The figure shows three views and two pictorial views of one solid part (mm, origin at its lowest corner). Answer the questions. A direction names the side the tool comes from. Round coordinates to 2 decimals unless told otherwise and drop trailing zeros. Order: outer loops, then holes, each group sorted by start corner. A loop starts at its lowest first (then second) coordinate and runs counter-clockwise, first axis right, second up. Notation, with made-up numbers: M 29,3.5 L 78,3.5 A13 ccw 78,17.5 Z; hole C 19.25,-32 d4. An arc over 180 degrees is marked long. Answer as CSV lines item,"result".
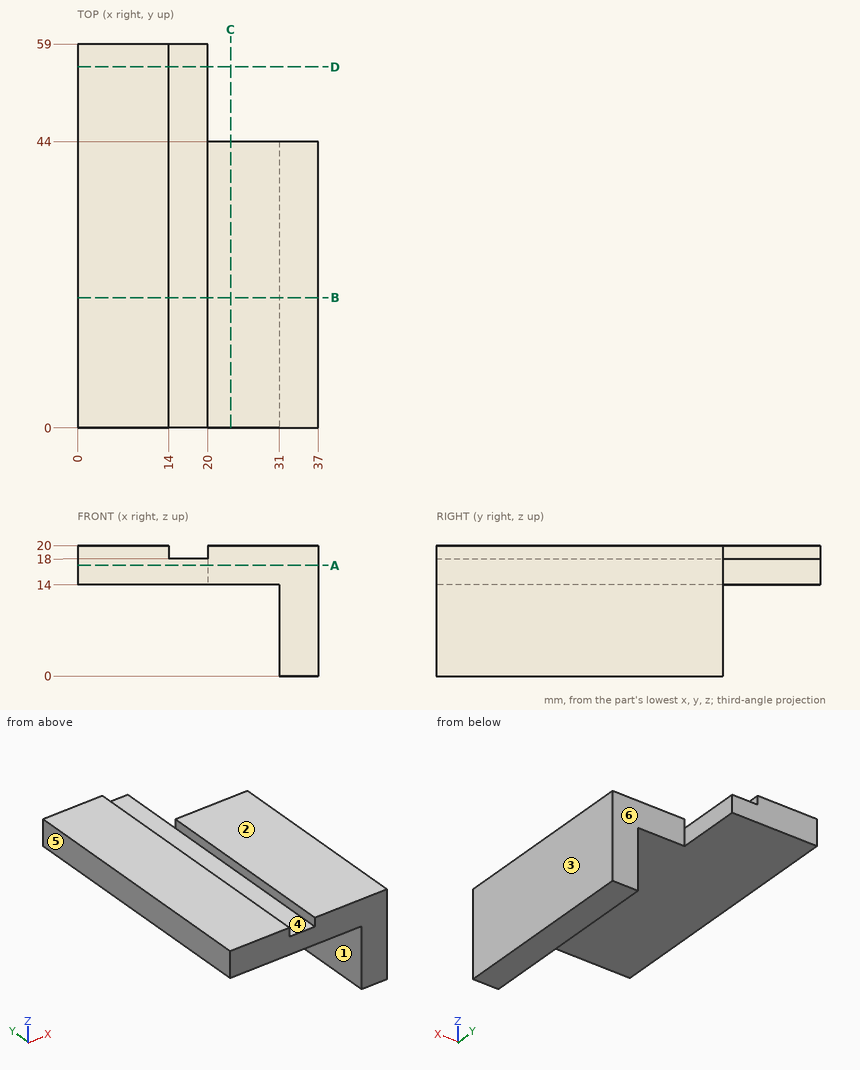
Item 1: Determine the mould class of the marked faces 3, 4, 5 and 6 for opening direction X: +X half, -X half, draft (parallel to the pull), parting line (faces both ways), or undercut.
Ans:
face 3,"+X half"
face 4,"undercut"
face 5,"-X half"
face 6,"draft"
Item 2: Flat-ended cylindrical pins translate along their axes: pin 1 (1.6 mm diameter, centred on y = 21.5, z = 18.5, fed in from -X); pin 2 (3 mm diameter, centred on x = 16, y = 20.5, fed in from +Z); pin 3 (8 mm diameter, centred on y = 29.5, z = 4, fed in from -X); pin 4 (1.2 mm diameter, centred on y = 49, z = 16, fed in from +X). Find the tip coordinate at first contact, or state that the pin passes through.
Ans:
pin 1,"x = 0"
pin 2,"z = 18"
pin 3,"x = 31"
pin 4,"x = 20"
Item 3: A cutting plane is placed at D-D, the plane y = 55.5. Determine the outline of the cut face in (x, z).
Ans:
outline,"M 0,14 L 20,14 L 20,18 L 14,18 L 14,20 L 0,20 Z"
Item 4: Find the intervals of material crossed by probe 1 along Z at (x, y) = (12, 35); probe 2 along Y at (x, z) = (33, 8.5); probe 3 along X at (y, z) = (39.5, 10), in increasing order. Write a range as [from, to].
Ans:
probe 1,"[14, 20]"
probe 2,"[0, 44]"
probe 3,"[31, 37]"
Item 5: A cutting plane is placed at C-C, the plane x = 23.5. Determine the outline of the cut face in (y, z), and give its area (3 significant figures).
Ans:
outline,"M 0,14 L 44,14 L 44,20 L 0,20 Z"
area,"264 mm2"
Item 6: A cutting plane is placed at B-B, the plane y = 20. Determine the outline of the cut face in (x, z).
Ans:
outline,"M 0,14 L 31,14 L 31,0 L 37,0 L 37,20 L 20,20 L 20,18 L 14,18 L 14,20 L 0,20 Z"
Item 7: A tool of negligible diameter and unlimited length cuts with its end or side. For the marked faces 1 and 2, from which of +Z, -Z, +X, -X, +Y, -Y can it reach the whole face along a straight path? Write none if from no direction.
Ans:
face 1,"-Z, -X, +Y, -Y"
face 2,"+Z, +X, -X, +Y, -Y"
Item 8: A cutting plane is placed at A-A, the plane z = 17. Determine the outline of the cut face in (x, y), and give its area (3 significant figures).
Ans:
outline,"M 0,0 L 37,0 L 37,44 L 20,44 L 20,59 L 0,59 Z"
area,"1,930 mm2"
